```python
from build123d import *

# Parameters (mm, degrees)
BOSS_EXTRUDE1_DEPTH = 2.5
BOSS_EXTRUDE2_DEPTH = 2.5
FILLET1_R           = 2
CUT_EXTRUDE1_DEPTH  = 34.176689588
BOSS_EXTRUDE3_DEPTH = 5


with BuildPart() as part:
    # Sketch1 → Boss-Extrude1 (new body)
    with BuildSketch(Plane(origin=(0, 0, 0), x_dir=(1, 0, 0), z_dir=(0, 1, 0))):
        with BuildLine():
            Line((-6.35, 0), (-6.35, -6.377891501))
            ThreePointArc((-6.35, -6.377891501), (0, 9), (6.35, -6.377891501))
            Line((6.35, -6.377891501), (6.35, 0))
            ThreePointArc((6.35, 0), (5.473649667, 4.068860406), (3, 7.416198487))
            ThreePointArc((3, 7.416198487), (0, 8), (-3, 7.416198487))
            ThreePointArc((-3, 7.416198487), (-5.473649667, 4.068860406), (-6.35, 0))
        make_face()
    extrude(amount=BOSS_EXTRUDE1_DEPTH)



with BuildPart() as body_2:
    # Sketch2 → Boss-Extrude2 (new body)
    with BuildSketch(Plane(origin=(0, 2.5, 0), x_dir=(1, 0, 0), z_dir=(0, 1, 0))):
        with BuildLine():
            Line((4.10424172, 11.276311449), (-15.426902632, 18.385066635))
            ThreePointArc((-15.426902632, 18.385066635), (-23.446511758, -5.124557191), (-6.35, -23.144707818))
            Line((-6.35, -23.144707818), (-6.35, -6.377891501))
            Line((-6.35, -6.377891501), (-6.35, 0))
            ThreePointArc((-6.35, 0), (-5.473649667, 4.068860406), (-3, 7.416198487))
            ThreePointArc((-3, 7.416198487), (0, 8), (3, 7.416198487))
            ThreePointArc((3, 7.416198487), (5.473649667, 4.068860406), (6.35, 0))
            Line((6.35, 0), (6.35, -10.182214887))
            ThreePointArc((6.35, -10.182214887), (11.934817997, 1.249047391), (4.10424172, 11.276311449))
        make_face()
    extrude(amount=BOSS_EXTRUDE2_DEPTH)

    # Fillet1
    fillet1_edges = [body_2.edges().sort_by_distance(p)[0] for p in [
        (-6.35, 3.75, 23.144707818),
        (-15.426902632, 3.75, -18.385066635),
    ]]
    fillet(fillet1_edges, radius=FILLET1_R)

    # Sketch3 → Cut-Extrude1 (cut, through all)
    with BuildSketch(Plane(origin=(0, 5, 0), x_dir=(1, 0, 0), z_dir=(0, 1, 0))):
        with BuildLine():
            ThreePointArc((-9.23213936, -16.834714219), (-8.717381687, -18.59965743), (-10.482324898, -19.114415103))
            ThreePointArc((-10.482324898, -19.114415103), (-21.553925967, -3.266232604), (-15.674771193, 15.150628635))
            ThreePointArc((-15.674771193, 15.150628635), (-13.836559277, 15.181884843), (-13.805303069, 13.343672927))
            ThreePointArc((-13.805303069, 13.343672927), (-18.983274246, -2.876681926), (-9.23213936, -16.834714219))
        make_face()
    extrude(amount=-CUT_EXTRUDE1_DEPTH, mode=Mode.SUBTRACT)


with BuildPart() as part_1:
    add(part.part)

    add(body_2.part)  # Boss-Extrude3 merges body 2
    # Sketch6 → Boss-Extrude3 (add)
    with BuildSketch(Plane(origin=(0, 5, 0), x_dir=(1, 0, 0), z_dir=(0, 1, 0))):
        with BuildLine():
            Line((6.35, -6.182214887), (6.35, -4.182214887))
            ThreePointArc((6.35, -4.182214887), (5.731966011, -5.182214887), (6.35, -6.182214887))
        make_face()
    boss_extrude3 = extrude(amount=-BOSS_EXTRUDE3_DEPTH)

    # Mirror1: Boss-Extrude3 across plane
    add(boss_extrude3.mirror(Plane(origin=(0, 0, 0), x_dir=(0, 0, 1), z_dir=(1, 0, 0))))


solid = part_1.part
```
CAD build for the part. Positions are in the model's coordinates, mm. A direction names the side the tool comes from. Round coordinates to 2 decimals unless told otherwise and drop trailing zeros. Write each loop counter-clockwise with the first axis right and the second up, starting at its lowest first coordinate (ties: lowest second). Pieces come first, ordered by that corner, then holes. Notation, with made-up numbers: (-3.5, 42.25) - (1.5, 42.25) arc R23 ccw to (1.5, 79.25) - close; hole circle Ø2 at (13.5, 13.25). An arc over 180 degrees is marked (long way). Write item = value, one per line. Start each with the question number.
Q1. Band-saw the part on C-C (z = -4). Give the cut face in (x, y), then the cut area to 3 significant figures.
Q2. Band-saw the part on B-B (x = -15). Give the cut face in (y, z) (3 decimals), then the cut area to 3 significant figures.
Q3. Drop flat-ended pins along their axis: pin 1 (1 mm diameter, centred on x = -17.5, y = 3.5, fed in from -Z); pin 2 (1.3 mm diameter, centred on y = 1.5, z = 2.5, fed in from +X); pin 3 (12 mm diameter, centred on x = -4, z = 17.5, fed in from -Y). Give the stop position or say it passes through.
Q4. Which spindle directions (+Z, -Z, +X, -X, +Y, -Y) get a long thin tool onto all of the face, cutting with end or side? Do faces 4 (the cylindrical face through (-5.732, 2.535, 5.165)), 5 (the cylindrical face through (-15.38, 3.77, -18.06)), 6 (the flat face through (6.35, 4, 8)), 7 (the cylindrical face through (0, 1, -9)). Say none if no direction does.
Q5. Mould opens along X. For faces 1 (the flat face through (-10, 5, -3)), 2 (the cylindrical face through (-21.51, 3.77, 3.54)), 3 (the cylindrical face through (11.953, 3.732, -1.062)) say: pulls with the +X half, pulls with the -X half, needs draft (parallel to the pull), parting line crosses it, or undercut.
Q6. Band-saw the part on D-D (y = 3.55). Give the cut face in (x, z), then the cut area to 3 significant figures.
Q7. Probe L1, parallel to Z at x = -16.5, y = 3.8; L2, parallel to X at y = 3.35, z = 5.5; L3, parallel to Y at x = -20, z = 12. List the from-to ranges inside material, lowest first. Write a range as from..to.
Q8. Band-saw the part on A-A (y = 1.45). Give the cut face in (x, z), then the cut area to 3 significant figures.
Answers below:
q1.outline = (-23.66, 2.5) - (-21.43, 2.5) - (-21.43, 5) - (-23.66, 5) - close; (-18.78, 2.5) - (-8.06, 2.5) - (-8.06, 0) - (-5.5, 0) - (-5.5, 5) - (-18.78, 5) - close; (5.5, 0) - (8.06, 0) - (8.06, 2.5) - (11.31, 2.5) - (11.31, 5) - (5.5, 5) - close
q1.area = 66.1 mm2
q2.outline = (2.5, -18.099) - (5, -18.099) - (5, -15.521) - (2.5, -15.521) - close; (2.5, -11.985) - (5, -11.985) - (5, 11.985) - (2.5, 11.985) - close; (2.5, 15.819) - (5, 15.819) - (5, 18.735) - (2.5, 18.735) - close
q2.area = 73.7 mm2
q3.pin_1 = -16.94
q3.pin_2 = 8.81
q3.pin_3 = 2.5
q4.face_4 = +Y, -Y
q4.face_5 = -Z, +Y, -Y
q4.face_6 = +Z, +Y, -Y
q4.face_7 = -Y
q5.face_1 = needs draft
q5.face_2 = undercut
q5.face_3 = pulls with the +X half
q6.outline = (-16.36, -17.56) arc R2 ccw to (-14.31, -17.98) - (4.1, -11.28) arc R12 ccw to (6.35, 10.18) - (6.35, 6.18) arc R1.12 ccw to (6.35, 4.18) - (6.35, 0) arc R9.88 cw to (3, -7.42) arc R8 cw to (-3, -7.42) arc R9.88 cw to (-6.35, 0) - (-6.35, 4.18) arc R1.12 ccw to (-6.35, 6.18) - (-6.35, 20.35) arc R2 ccw to (-9.11, 22.2) arc R24 ccw to start; hole (-15.67, -15.15) arc R1.3 ccw to (-13.81, -13.34) arc R19.2 cw to (-9.23, 16.83) arc R1.3 ccw to (-10.48, 19.11) arc R21.8 ccw to start
q6.area = 622 mm2
q7.L1 = -17.43..-14.25, -9.82..9.82, 14.25..17.43
q7.L2 = -23.36..-21.09, -18.4..-5.78, 5.78..10.67
q7.L3 = 2.5..5
q8.outline = (-6.35, 0) - (-6.35, 4.18) arc R1.12 ccw to (-6.35, 6.18) - (-6.35, 6.38) arc R9 ccw (long way) to (6.35, 6.38) - (6.35, 6.18) arc R1.12 ccw to (6.35, 4.18) - (6.35, 0) arc R9.88 cw to (3, -7.42) arc R8 cw to (-3, -7.42) arc R9.88 cw to start
q8.area = 71.0 mm2
